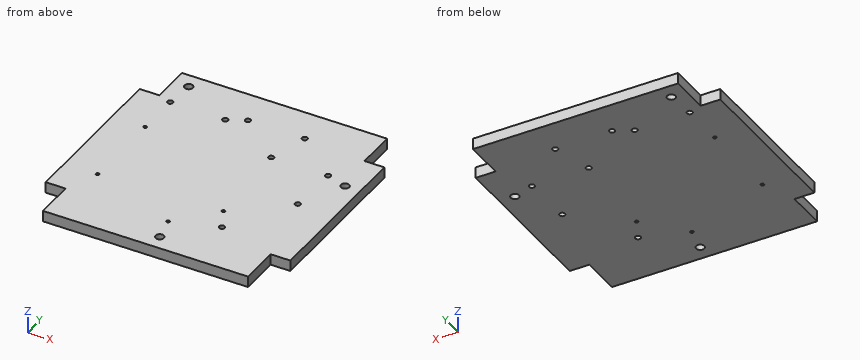
```python
from build123d import *

# Parameters (mm, degrees)
SZKIC2_R                    = 0.75
SZKIC2_R_2                  = 1.875
SZKIC2_R_3                  = 1.25
DODANIE_WYCI_GNI_CIE1_DEPTH = 5


with BuildPart() as part:
    # Szkic2 → Dodanie-wyciągnięcie1 (new body)
    with BuildSketch(Plane.XY):
        Polygon((9, 18), (9, 0), (102, 0), (102, 18), (111, 18), (111, 93), (102, 93), (102, 111), (9, 111), (9, 93), (0, 93), (0, 18), align=None)
        with Locations((15, 33)):
            Circle(SZKIC2_R, mode=Mode.SUBTRACT)
        with Locations((58, 7)):
            Circle(SZKIC2_R_2, mode=Mode.SUBTRACT)
        with Locations((55.5, 18)):
            Circle(SZKIC2_R, mode=Mode.SUBTRACT)
        with Locations((76, 25)):
            Circle(SZKIC2_R_3, mode=Mode.SUBTRACT)
        with Locations((71, 35)):
            Circle(SZKIC2_R, mode=Mode.SUBTRACT)
        with Locations((94, 53.844410204)):
            Circle(SZKIC2_R_3, mode=Mode.SUBTRACT)
        with Locations((15, 71)):
            Circle(SZKIC2_R, mode=Mode.SUBTRACT)
        with Locations((15, 91)):
            Circle(SZKIC2_R_3, mode=Mode.SUBTRACT)
        with Locations((16, 104)):
            Circle(SZKIC2_R_2, mode=Mode.SUBTRACT)
        with Locations((40, 91)):
            Circle(SZKIC2_R_3, mode=Mode.SUBTRACT)
        with Locations((48, 95)):
            Circle(SZKIC2_R_3, mode=Mode.SUBTRACT)
        with Locations((68.790622886, 77)):
            Circle(SZKIC2_R_3, mode=Mode.SUBTRACT)
        with Locations((94.581245773, 77)):
            Circle(SZKIC2_R_3, mode=Mode.SUBTRACT)
        with Locations((104, 74)):
            Circle(SZKIC2_R_2, mode=Mode.SUBTRACT)
        with Locations((73.790622886, 95)):
            Circle(SZKIC2_R_3, mode=Mode.SUBTRACT)
    extrude(amount=DODANIE_WYCI_GNI_CIE1_DEPTH)


solid = part.part
```
The listing builds one solid part. Answer for the finished solid, in the listing's coordinates (mm). Coordinates: 2 decimals unless noted, no trailing zeros. Loops run counter-clockwise (first coordinate to the right, second up) from the corner with the lowest first, then second, coordinate; pieces in that order, holes last. Notation, with made-up numbers: M 24,84 L 53,84 A24 cw 53,98 Z; hole C -33.75,-5 d8. An arc over 180 degrees is marked long. Answer as a JSON object with one key per item and string values. Group by question number.
Item 1: Section C-C (z = 2.8) is taken. Give the number of separate pieces and of enclosed holes in the cut face, and give its area (3 significant figures).
Item 2: Each of these flat-tipped pins is pushed along its axis until it touches: P1, Ø2.5, axis at x = 15, y = 71, coming from the +Z side; P2, Ø3.5, axis at x = 58, y = 7, coming from the -Z side; P3, Ø2.5, axis at y = 4.5, z = 2, coming from the -X side; P4, Ø1.5, axis at y = 105.5, z = 3.5, coming from the +X side. Where does it stop, or does it pass through?
Item 3: Section B-B (x = 58) is taken. Write down the section's boundary in (y, z) (3 decimals), and give its area (3 significant figures).
Item 4: Consider L1, parallel to X at y = 95, z = 3.5; L2, parallel to X at y = 91, z = 3.55; L3, parallel to Y at x = 71, z = 2.45. Determine where each line is inside the solid, lowest interval first.
Item 5: Section A-A (y = 7) is taken. Write down the section's boundary in (x, z) (3 decimals).
Solved:
{
 "1": {"separate pieces": "1", "enclosed holes": "15", "area": "11,600 mm2"},
 "2": {"P1": "stops at z = 5", "P2": "passes through", "P3": "stops at x = 9", "P4": "stops at x = 102"},
 "3": {"outline": "M 0,0 L 5.125,0 L 5.125,5 L 0,5 Z; M 8.875,0 L 111,0 L 111,5 L 8.875,5 Z", "area": "536 mm2"},
 "4": {"L1": "x = 9 to 46.75, 49.25 to 72.54, 75.04 to 102", "L2": "x = 0 to 13.75, 16.25 to 38.75, 41.25 to 111", "L3": "y = 0 to 34.25, 35.75 to 111"},
 "5": {"outline": "M 9,0 L 56.125,0 L 56.125,5 L 9,5 Z; M 59.875,0 L 102,0 L 102,5 L 59.875,5 Z"}
}
